The model under review builds one solid part; all positions refer to its coordinate system, in mm. Face numbers are marked on the shaded views. A direction names the side the tool comes from. Give positions to 0.01 mm unless a question says otherwise; leave off trailing zeros. Write each loop counter-clockwise with the first axis right and the second up, starting at its lowest first coordinate (ties: lowest second). Pieces come first, ordered by that corner, then holes. Notation, with made-up numbers: M 56,0 L 98,0 A30 cw 98,32 Z; hole C 14,29 d4. An arc over 180 degrees is marked long. Write item = value, one per line. Start each with the question number.
```python
from build123d import *

# Parameters (mm, degrees)
SKETCH_1_R          = 18
EXTRUDE_1_DEPTH     = 43.573
SKETCH_3_R          = 25.5
SKETCH_3_R_2        = 2.1
EXTRUDE_2_DEPTH     = 7
SKETCH_2_R          = 2
CUT_EXTRUDE_1_DEPTH = 10


with BuildPart() as part:
    # Эскиз1 → Бобышка-Вытянуть1 (new body)
    with BuildSketch(Plane(origin=(0, 0, 0), x_dir=(1, 0, 0), z_dir=(0, 1, 0))):
        with Locations(Location((0, 0, 0), (0, 0, 270))):
            Circle(SKETCH_1_R)
    extrude(amount=EXTRUDE_1_DEPTH)

    # Эскиз3 → Бобышка-Вытянуть2 (add)
    with BuildSketch(Plane.XZ):
        with Locations(Location((0, 0, 0), (0, 0, 270))):
            Circle(SKETCH_3_R)
        with Locations(Location((0, 22, 0), (0, 0, 270))):
            Circle(SKETCH_3_R_2, mode=Mode.SUBTRACT)
        with Locations(Location((-22, 0, 0), (0, 0, 270))):
            Circle(SKETCH_3_R_2, mode=Mode.SUBTRACT)
        with Locations(Location((0, -22, 0), (0, 0, 270))):
            Circle(SKETCH_3_R_2, mode=Mode.SUBTRACT)
        with Locations(Location((22, 0, 0), (0, 0, 270))):
            Circle(SKETCH_3_R_2, mode=Mode.SUBTRACT)
    extrude(amount=-EXTRUDE_2_DEPTH)

    # Эскиз2 → Вырез-Вытянуть1 (cut)
    with BuildSketch(Plane(origin=(0, 43.573, 0), x_dir=(1, 0, 0), z_dir=(0, 1, 0))):
        with Locations(Location((0.008308586, 14.359840693, 0), (0, 0, 270))):
            Circle(SKETCH_2_R)
        with Locations(Location((13.669247008, -4.399634075, 0), (0, 0, 270))):
            Circle(SKETCH_2_R)
        with Locations(Location((0.018947935, -14.359830595, 0), (0, 0, 270))):
            Circle(SKETCH_2_R)
        with Locations(Location((-13.677573358, 4.373680464, 0), (0, 0, 270))):
            Circle(SKETCH_2_R)
    extrude(amount=-CUT_EXTRUDE_1_DEPTH, mode=Mode.SUBTRACT)


solid = part.part
```
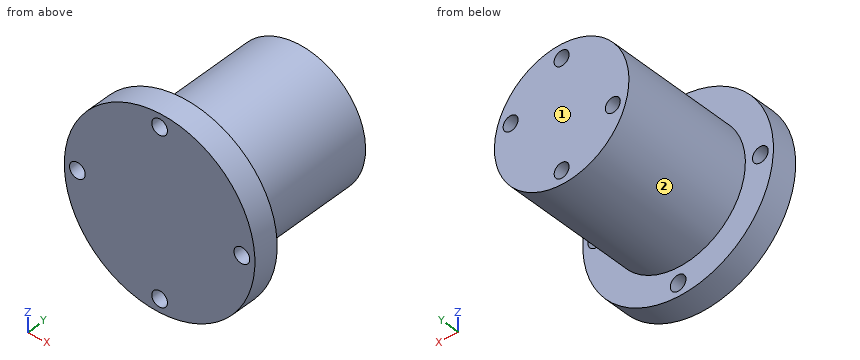
Item 1: For the marked faces 1 and 2, list the 3-axis set-ups (+Z, -Z, +X, -X, +Y, -Y) from which the entire face can be reached by the end or side of a thin tool; tool diameter is ignored.
Item 2: We need section D-D, the plane x = 21. Write out the cut boundary in (y, z).
Item 3: We need section A-A, the plane z = 22. Write out the cut boundary in (x, y).
Item 4: Clearance check with flat-ended pins moving along their axes: P1, Ø1.2, axis at x = -13, z = -5.5, coming from the +Y side; P2, Ø3.5, axis at x = 0.02, z = 14.36, coming from the -Y side; P3, Ø8, axis at y = 32, z = 0, coming from the -X side; P4, Ø6.5, axis at x = 22, z = 0, coming from the +Y side. State where each tip first meets the part, or that it passes through.
Item 5: We need section C-C, the plane x = 1. Write out the cut boundary in (y, z), and give its area (3 significant figures).
Item 6: To check wall thickness, follow probe 1 along Y at (x, z) = (-18, -9.5); probe 2 along X at (y, z) = (38.5, -16); probe 3 along Z at (x, y) = (-13, 41.5). State the ranges of each line that lie inside material, in increasing order. Write a range as [from, to].
Item 7: We need section B-B, the plane y = 5.5. Write out the cut boundary in (x, z).
Worked out:
q1.face_1 = +Z, -Z, +X, -X, +Y
q1.face_2 = +Y
q2.outline = M 0,-14.47 L 7,-14.47 L 7,-1.85 L 0,-1.85 Z; M 0,1.85 L 7,1.85 L 7,14.47 L 0,14.47 Z
q3.outline = M -12.89,0 L -2.1,0 L -2.1,7 L -12.89,7 Z; M 2.1,0 L 12.89,0 L 12.89,7 L 2.1,7 Z
q4.P1 = 33.57
q4.P2 = 0
q4.P3 = -18
q4.P4 = 7
q5.outline = M 0,-25.48 L 7,-25.48 L 7,-23.85 L 0,-23.85 Z; M 0,-20.15 L 7,-20.15 L 7,-17.97 L 43.57,-17.97 L 43.57,-16.1 L 33.57,-16.1 L 33.57,-12.62 L 43.57,-12.62 L 43.57,12.62 L 33.57,12.62 L 33.57,16.1 L 43.57,16.1 L 43.57,17.97 L 7,17.97 L 7,20.15 L 0,20.15 Z; M 0,23.85 L 7,23.85 L 7,25.48 L 0,25.48 Z
q5.area = 1,550 mm²
q6.probe_1 = [0, 7]
q6.probe_2 = [-8.25, -1.14], [1.15, 8.25]
q6.probe_3 = [-12.45, -6.26], [-2.49, 12.45]
q7.outline = C 0,0 d51; hole C -22,0 d4.2; hole C 0,-22 d4.2; hole C 0,22 d4.2; hole C 22,0 d4.2
